Can you work these out from the model? Positions are in its coordinate system, mm. Face numbers are marked on the shaded views. Coordinates: 2 decimals unless noted, no trailing zeros. Order: outer loops, then holes, each group sorted by start corner. A loop starts at its lowest first (then second) coordinate and runs counter-clockwise, first axis right, second up. Notation, with made-up numbers: (-32.5, 52.25) -> (-24.5, 52.25) arc R24 ccw to (-24.5, 75.25) -> close; hole circle Ø5 at (12, 75.5). An arc over 180 degrees is marked (long way). Write item = value, one per line. Start each with the question number.
from build123d import *

# Parameters (mm, degrees)
SKETCH_R    = 4
PAD_DEPTH   = 10
FILLET_R    = 7
FILLET001_R = 162
FILLET002_R = 4


with BuildPart() as part:
    # Sketch → Pad (new body)
    with BuildSketch(Plane.XY):
        Polygon((-75, -20), (-75, 0), (75, 0), (75, -20), (93, -20), (85, 10), (60, 5), (-60, 5), (-85, 10), (-85, -20), align=None)
        with Locations((83, -12)):
            Circle(SKETCH_R, mode=Mode.SUBTRACT)
    extrude(amount=PAD_DEPTH)

    # Fillet
    fillet_edges = [part.edges().sort_by_distance(p)[0] for p in [
        (85, 10, 5),
        (-85, 10, 5),
    ]]
    fillet(fillet_edges, radius=FILLET_R)

    # Fillet001
    fillet001_edges = [part.edges().sort_by_distance(p)[0] for p in [
        (-60, 5, 5),
        (60, 5, 5),
    ]]
    fillet(fillet001_edges, radius=FILLET001_R)

    # Fillet002
    fillet002_edges = [part.edges().sort_by_distance(p)[0] for p in [
        (93, -20, 5),
    ]]
    fillet(fillet002_edges, radius=FILLET002_R)


solid = part.part
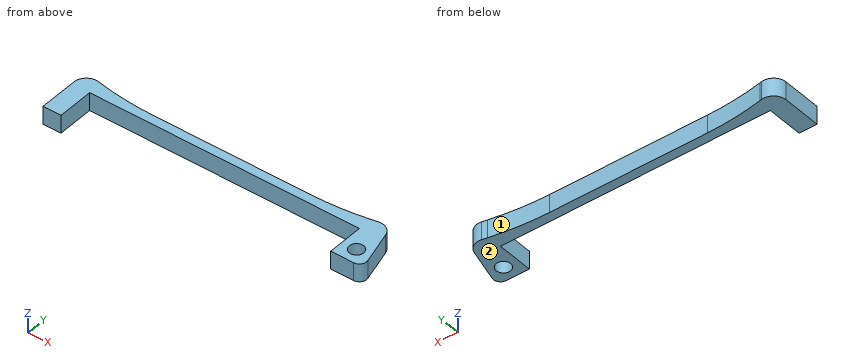
(1) Imagine slicing it at D-D (x = -18). Write out the boundary of the cut face in (y, z).
(2) Imagine slicing it at A-A (x = 83). Write out the boundary of the cut face in (y, z), plus the area to 3 significant figures.
(3) If I drill on L1, parallel to X at y = -12.75, z = 9; L2, parallel to Y at x = 83, z = 6; L3, parallel to Y at x = -31.5, z = 5.5, over which ranges is the centre line in solid material (lowest first)? Write a range as from..to.
(4) For P1, Ø2, axis at x = -23.5, z = 4.5, coming from the -Y side; P2, Ø10, axis at x = 72, y = 1, coming from the -Z side; P3, Ø6, axis at x = 35.5, z = 7.5, coming from the +Y side; P4, Ø5, axis at y = -6.5, z = 6, coming from the +X side, each with a flat end and sliding along its axis, tell me the tip position at first contact or that it passes through.
(5) Thinking about a two-plate mould opening in X: for the marked faces 1 and 2, which applies, +X half, -X half, draft (parallel to the pull), parting line (faces both ways), or undercut?
(6) Imagine slicing it at B-B (z = 3.25). Write out the boundary of the cut face in (x, y), plus the area to 3 significant figures.
(7) Imagine slicing it at C-C (y = -6). Write out the boundary of the cut face in (x, z), plus the area to 3 significant figures.
Result set:
q1.outline = (0, 0) -> (5, 0) -> (5, 10) -> (0, 10) -> close
q2.outline = (-20, 0) -> (-16, 0) -> (-16, 10) -> (-20, 10) -> close; (-8, 0) -> (8.14, 0) -> (8.14, 10) -> (-8, 10) -> close
q2.area = 201 mm2
q3.L1 = -85..-75, 75..79.07, 86.93..91.07
q3.L2 = -20..-16, -8..8.14
q3.L3 = 0..5
q4.P1 = 0
q4.P2 = 0
q4.P3 = 5
q4.P4 = 90.07
q5.face_1 = undercut
q5.face_2 = draft
q6.outline = (-85, -20) -> (-75, -20) -> (-75, 0) -> (75, 0) -> (75, -20) -> (87.79, -20) arc R4 ccw to (91.66, -14.97) -> (86.69, 3.65) arc R7 ccw to (78.56, 8.71) -> (75.73, 8.15) arc R162 cw to (43.96, 5) -> (-43.96, 5) arc R162 cw to (-75.73, 8.15) -> (-76.63, 8.33) arc R7 ccw to (-85, 1.46) -> close; hole circle Ø8 at (83, -12)
q6.area = 1,430 mm2
q7.outline = (-85, 0) -> (-75, 0) -> (-75, 10) -> (-85, 10) -> close; (75, 0) -> (89.27, 0) -> (89.27, 10) -> (75, 10) -> close
q7.area = 243 mm2
